The listing builds one solid part. Answer for the finished solid, in the listing's coordinates (mm). Face numbers are marked on the shaded views. A direction names the side the tool comes from. Round coordinates to 2 decimals unless told otherwise and drop trailing zeros. Order: outer loops, then holes, each group sorted by start corner. A loop starts at its lowest first (then second) coordinate and runs counter-clockwise, first axis right, second up. Notation, with made-up numbers: (-37, 7.25) -> (0, 7.25) arc R16 cw to (0, 35.25) -> close; hole circle Ø3 at (53.25, -31). An arc over 180 degrees is marked (long way). Return JSON: item names as keys, results as strings. Group by question number.
(1) Determine the mould class of the marked faces 4, 5 and 6 for opening direction Z: +Z half, -Z half, draft (parallel to the pull), parting line (faces both ways), or undercut.
(2) The part is cut by section A-A (x = -35.5). Determine the outline of the cut face in (y, z), plus the area to 3 significant figures.
(3) The part is cut by section B-B (z = -88). Determine the outline of the cut face in (x, y), plus the area to 3 significant figures.
(4) Which of the six approach directions +Z, -Z, +X, -X, +Y, -Y give full straight-line access (tool end or side, diameter ignored) to the marked faces 1, 2 and 3?
(5) This flat-tipped pin is pushed along its axis until it touches: pin 1 (11.5 mm diameter, centred on y = 15.5, z = -93, fed in from -X). Where does it stop, or does it pass through?
(6) The part is cut by section D-D (x = -28). Determine the outline of the cut face in (y, z), plus the area to 3 significant figures.
(7) Consider line 1 (Z direction, x = -9.5, y = 57); line 2 (X direction, y = 20.5, z = -81); line 3 (Z direction, x = -46, y = 6.5). Determine where each line is inside the solid, lowest interval first. Write a range as [from, to].
(8) The part is cut by section C-C (y = 24.5). Determine the outline of the cut face in (x, z), plus the area to 3 significant figures.
Autodesk Inventor part; units mm, degrees
ref_plane "YZ Plane" through (0, 0, 0) normal (1, 0, 0) x (0, 1, 0)
ref_plane "XZ Plane" through (0, 0, 0) normal (0, 1, 0) x (-1, 0, 0)
ref_plane "XY Plane" through (0, 0, 0) normal (0, 0, 1) x (1, 0, 0)
sketch "Sketch1" plane through (0, 0, 0) normal (0, 1, 0) x (-1, 0, 0)
  line L0 (0, 0) -> (25.4, 0)
  line L1 (25.4, 0) -> (25.4, -127)
  line L2 (25.4, -127) -> (0, -127)
  line L3 (0, -127) -> (0, 0)
  line L4 (30.48, 5.08) -> (-5.08, 5.08)
  line L5 (-5.08, 5.08) -> (-5.08, -132.08)
  line L6 (-5.08, -132.08) -> (30.48, -132.08)
  line L7 (30.48, -132.08) -> (30.48, 5.08)
  dimension "d0" = 25.4
  dimension "d1" = 127
  dimension "d2" = 5.08
  dimension "d3" = 5.08
  dimension "d4" = 5.08
  dimension "d5" = 5.08
extrude "Extrusion1" add sketch "Sketch1" along normal blind 38.1
sketch "Sketch2" plane through (0, 38.1, 0) normal (0, 1, 0) x (1, 0, 0)
  line L0 (-30.48, -5.08) -> (5.08, -5.08)
  line L1 (5.08, -5.08) -> (-62.5812, -5.08)
  line L2 (-62.5812, -5.08) -> (-62.5812, 0)
  line L3 (-62.5812, 0) -> (0, 0)
  line L4 (-25.4, 127) -> (0, 127)
  line L5 (0, 127) -> (-62.5812, 127)
  line L6 (5.08, -5.08) -> (5.08, 132.08)
  line L7 (5.08, -5.08) -> (-62.5812, -5.08)
  line L8 (-62.5812, 132.08) -> (5.08, 132.08)
  line L9 (5.08, 132.08) -> (5.08, -5.08)
  line L10 (-62.5812, 132.08) -> (-47.0844, 132.08)
  line L11 (-62.5812, 127) -> (-62.5812, 132.08)
  line L12 (0, 127) -> (0, 0)
  line L13 (0, 0) -> (0, 127)
  line L14 (0, 127) -> (-62.5812, 127)
  line L15 (-62.5812, 132.08) -> (3.2473, 132.08)
  line L16 (5.08, 132.08) -> (-30.48, 132.08)
extrude "Extrusion2" add sketch "Sketch2" along normal blind 25.4
sketch "Sketch5" plane through (0, 38.1, 0) normal (0, -1, 0) x (1, 0, 0)
  line L0 (-62.5812, -132.08) -> (-62.5812, -127)
  line L1 (-30.48, -132.08) -> (-30.48, 5.08)
  line L2 (-62.5812, -132.08) -> (-30.48, -132.08)
  line L3 (-30.48, -132.08) -> (-30.48, -126.7104)
  line L4 (-30.48, -126.7104) -> (-62.5812, -126.7104)
  line L5 (-62.5812, -126.7104) -> (-62.5812, -132.08)
  line L6 (-62.5812, 0) -> (-62.5812, 5.08)
  line L7 (-30.48, 5.08) -> (5.08, 5.08)
  line L8 (-62.5812, 0) -> (-30.48, 0)
  line L9 (-30.48, 0) -> (-30.48, 5.08)
  line L10 (-30.48, 5.08) -> (-62.5812, 5.08)
  line L11 (-62.5812, 5.08) -> (-62.5812, 0)
  point P0 (0, 0)
extrude "Extrusion3" add sketch "Sketch5" along normal blind 38.1
properties part number "Base2"
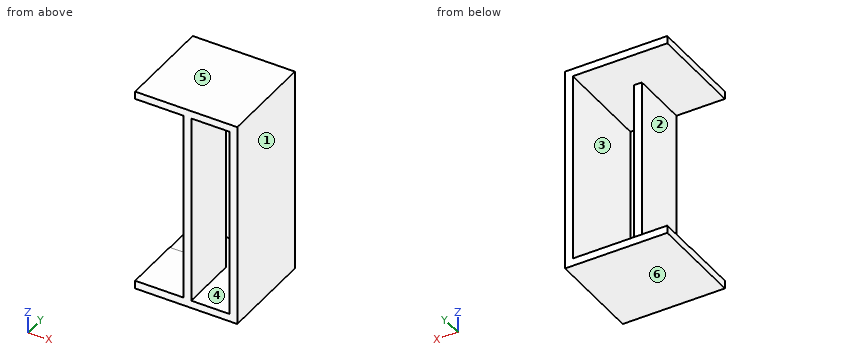
Answer below:
{
 "1": {"face 4": "undercut", "face 5": "+Z half", "face 6": "-Z half"},
 "2": {"outline": "(0, -132.08) -> (63.5, -132.08) -> (63.5, -127) -> (38.1, -127) -> (38.1, -126.71) -> (0, -126.71) -> close; (0, 0) -> (63.5, 0) -> (63.5, 5.08) -> (0, 5.08) -> close", "area": "656 mm²"},
 "3": {"outline": "(-30.48, 0) -> (-25.4, 0) -> (-25.4, 38.1) -> (-30.48, 38.1) -> close; (0, 0) -> (5.08, 0) -> (5.08, 63.5) -> (0, 63.5) -> close", "area": "516 mm²"},
 "4": {"face 1": "+Z, -Z, +X, +Y, -Y", "face 2": "-X, +Y, -Y", "face 3": "+Y, -Y"},
 "5": {"pin 1": "stops at x = -30.48"},
 "6": {"outline": "(0, -132.08) -> (63.5, -132.08) -> (63.5, -127) -> (38.1, -127) -> (38.1, 0) -> (63.5, 0) -> (63.5, 5.08) -> (0, 5.08) -> close", "area": "5,480 mm²"},
 "7": {"line 1": "z = [-132.08, -127], [0, 5.08]", "line 2": "x = [-30.48, -25.4], [0, 5.08]", "line 3": "z = [-132.08, -126.71], [0, 5.08]"},
 "8": {"outline": "(-62.58, -132.08) -> (5.08, -132.08) -> (5.08, 5.08) -> (-62.58, 5.08) -> (-62.58, 0) -> (-30.48, 0) -> (-30.48, -126.71) -> (-62.58, -126.71) -> close; hole (-25.4, -127) -> (0, -127) -> (0, 0) -> (-25.4, 0) -> close", "area": "1,990 mm²"}
}
